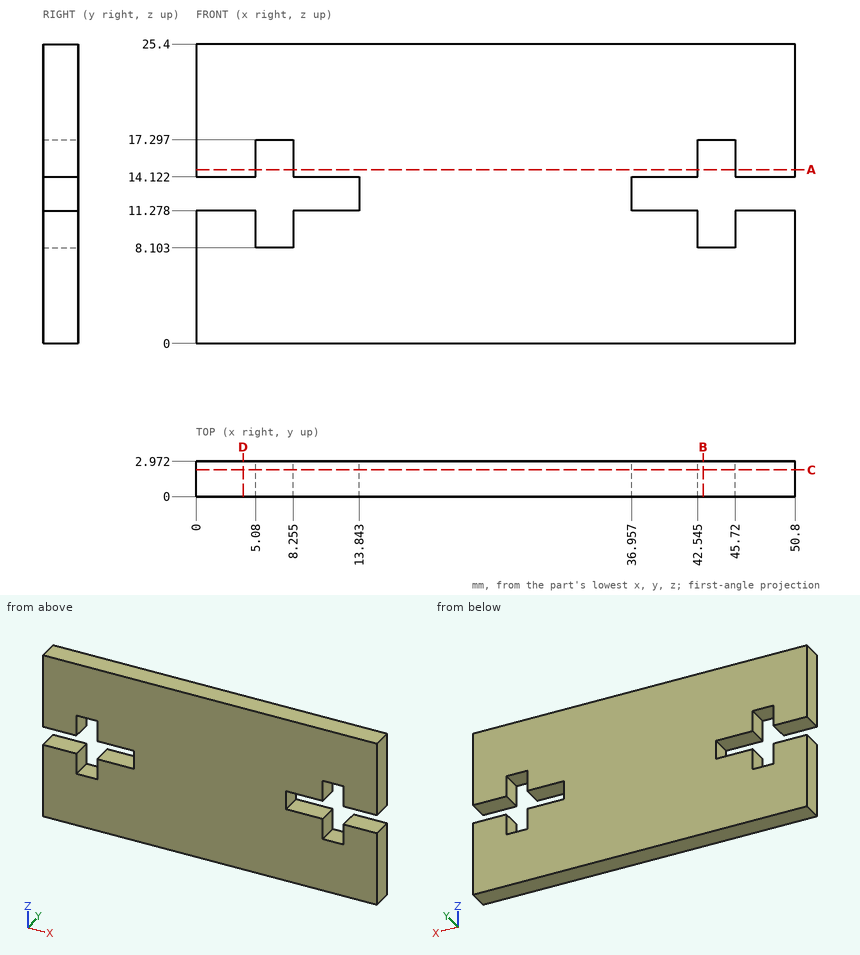
Geometry check sheet. Reference: drawing and pictorial views, mm from the part's lowest x, y, z. Round coordinates to 2 decimals unless told otherwise and drop trailing zeros. Loops run counter-clockwise (first coordinate to the right, second up) from the corner with the lowest first, then second, coordinate; pieces in that order, holes last. Notation, with made-up numbers: (26, 40) - (58, 40) arc R11 cw to (58, 60) - close; hole circle Ø6 at (-17.75, -15.5). An arc over 180 degrees is marked (long way). Use a Markdown table: item, result.
Q1. Go/stop test with a flat-tipped pin: P1, Ø0.9, axis at y = 0.5, z = 9, coming from the -X side. Record where the tip stops, or that it passes through.
Solutions:
| item | result |
|---|---|
| P1 | stops at x = 0 |
Q2. Cross-section at D-D on x = 4. Record the cut outline in (y, z).
Solutions:
| item | result |
|---|---|
| outline | (0, 0) - (2.97, 0) - (2.97, 11.28) - (0, 11.28) - close; (0, 14.12) - (2.97, 14.12) - (2.97, 25.4) - (0, 25.4) - close |
Q3. Cross-section at A-A on z = 14.75. Record the cut outline in (x, y) (1 decimal).
Solutions:
| item | result |
|---|---|
| outline | (0, 0) - (5.1, 0) - (5.1, 3) - (0, 3) - close; (8.3, 0) - (42.5, 0) - (42.5, 3) - (8.3, 3) - close; (45.7, 0) - (50.8, 0) - (50.8, 3) - (45.7, 3) - close |
Q4. Material ranges on line 1 (X direction, y = 2.1, z = 16) (1 decimal); line 2 (Z direction, x = 43, y = 2.3); line 3 (Z direction, x = 48, y = 1.7), recorded low to high.
Solutions:
| item | result |
|---|---|
| line 1 | x = 0 to 5.1, 8.3 to 42.5, 45.7 to 50.8 |
| line 2 | z = 0 to 8.1, 17.3 to 25.4 |
| line 3 | z = 0 to 11.28, 14.12 to 25.4 |
Q5. Cross-section at C-C on y = 2.25. Record the cut outline in (x, z) (1 decimal), plus the area to 3 significant figures.
Solutions:
| item | result |
|---|---|
| outline | (0, 0) - (50.8, 0) - (50.8, 11.3) - (45.7, 11.3) - (45.7, 8.1) - (42.5, 8.1) - (42.5, 11.3) - (37, 11.3) - (37, 14.1) - (42.5, 14.1) - (42.5, 17.3) - (45.7, 17.3) - (45.7, 14.1) - (50.8, 14.1) - (50.8, 25.4) - (0, 25.4) - (0, 14.1) - (5.1, 14.1) - (5.1, 17.3) - (8.3, 17.3) - (8.3, 14.1) - (13.8, 14.1) - (13.8, 11.3) - (8.3, 11.3) - (8.3, 8.1) - (5.1, 8.1) - (5.1, 11.3) - (0, 11.3) - close |
| area | 1,170 mm2 |
Q6. Cross-section at B-B on x = 43. Record the cut outline in (y, z).
Solutions:
| item | result |
|---|---|
| outline | (0, 0) - (2.97, 0) - (2.97, 8.1) - (0, 8.1) - close; (0, 17.3) - (2.97, 17.3) - (2.97, 25.4) - (0, 25.4) - close |
